Build history of the part. All positions in model axes, mm. A direction names the side the tool comes from. Coordinates: 2 decimals unless noted, no trailing zeros. Loops run counter-clockwise (first coordinate to the right, second up) from the corner with the lowest first, then second, coordinate; pieces in that order, holes last.
Item 1: Mould opens along Z. For faces 1 (the face through (6, 0, -1)), 2 (the face through (3.042, 14.012, 8.536)), 3 (the face through (2.949, 0.459, -34.887)), 4 (the face through (3, 0, -5)) say: released by +Z, released by -Z, zero draft, split by the parting line, or undercut.
Item 2: Cut at A-A (y = -14.5). List the corners of the cut face in (x, z), and give its area (3 significant figures).
Item 3: 3-axis set-ups, long thin cutter, end or side, ignore diameter. For faces 5 (the face through (0, 16, -42)), 6 (the face through (3, 0, -30)), 7 (the face through (0, -13, 1)), 8 (the face through (0, 16, 7)): which of +Z, -Z, +X, -X, +Y, -Y reach the whole face in a straight line?
Item 4: Flat gauge pins, fed straight in: pin 1 (2 mm diameter, centred on x = -6, y = -10, fed in from -Z); pin 2 (6.5 mm diameter, centred on y = 14.5, z = 4, fed in from +X); pin 3 (1 mm diameter, centred on x = -1, y = -14, fed in from +Z); pin 4 (3 mm diameter, centred on y = 4.5, z = -4, fed in from -X). Where does each tip first touch, or does it go through?
Item 5: Drill centre lines: line 1 along Y through (x, z) = (3.6, 4); line 2 along Y through (x, z) = (-13.5, -15); line 3 along Z through (x, y) = (-4.25, -4.5). Where is each one in solid material? Low to high.
from build123d import *

# Parameters (mm, degrees)
BOSS_EXTRUDE2_DEPTH      = 21.5
CUT_EXTRUDE8_DEPTH       = 44
CUT_EXTRUDE9_DEPTH       = 24.5
SKETCH18_R               = 2.5
CUT_EXTRUDE13_DEPTH      = 18.5000001
CUT_EXTRUDE13_DEPTH_BACK = 7.0000001
SKETCH19_RX              = 11.071840333
SKETCH19_RY              = 5.954349413
CUT_EXTRUDE14_DEPTH      = 7.0000001
CUT_EXTRUDE14_DEPTH_BACK = 18.5000001
FILLET6_R                = 2
FILLET7_R                = 2


with BuildPart() as part:
    # Sketch12 → Boss-Extrude2 (new body, symmetric)
    with BuildSketch(Plane(origin=(0, 0, 0), x_dir=(1, 0, 0), z_dir=(0, 1, 0))):
        with BuildLine():
            Line((0, 35), (0, 52))
            Line((0, 52), (6, 52))
            Line((6, 52), (6, -17))
            Line((6, -17), (0, -17))
            Line((0, -17), (0, 0))
            ThreePointArc((0, 0), (-17.5, 17.5), (0, 35))
        make_face()
    extrude(amount=BOSS_EXTRUDE2_DEPTH, both=True)

    # Sketch13 → Cut-Extrude8 (cut, through all)
    with BuildSketch(Plane.XZ.offset(21.5)):
        with BuildLine():
            Line((0, -30), (6, -30))
            Line((6, -30), (6, -5))
            Line((6, -5), (0, -5))
            ThreePointArc((0, -5), (-12.5, -17.5), (0, -30))
        make_face()
    extrude(amount=-CUT_EXTRUDE8_DEPTH, mode=Mode.SUBTRACT)

    # Sketch14 → Cut-Extrude9 (cut, through all)
    with BuildSketch(Plane(origin=(6, 0, 0), x_dir=(0, 0, -1), z_dir=(1, 0, 0))):
        with BuildLine():
            Line((-3.475, -21.5), (-17, -21.5))
            Line((-17, -21.5), (-17, 21.5))
            Line((-17, 21.5), (-5.475, 21.5))
            ThreePointArc((-5.475, 21.5), (-8.517618353, 13.892451617), (-3.272109233, 7.598251675))
            ThreePointArc((-3.272109233, 7.598251675), (0.112562803, 0.342782413), (-3.475, -6.814537766))
            ThreePointArc((-3.475, -6.814537766), (-8.299421353, -14.157268883), (-3.475, -21.5))
        make_face()
    cut_extrude9 = extrude(amount=-CUT_EXTRUDE9_DEPTH, mode=Mode.SUBTRACT)

    # Mirror1: Cut-Extrude9 across plane
    add(cut_extrude9.mirror(Plane.XY.offset(-17.5)), mode=Mode.SUBTRACT)

    # Sketch18 → Cut-Extrude13 (cut, two sides)
    with BuildSketch(Plane.ZY) as cut_extrude13_sk:
        with Locations((-39, 14.5)):
            Circle(SKETCH18_R)
        with Locations((4, 14.5)):
            Circle(SKETCH18_R)
        with Locations((-39, -14.5)):
            Circle(SKETCH18_R)
        with Locations((4, -14.5)):
            Circle(SKETCH18_R)
    extrude(amount=CUT_EXTRUDE13_DEPTH, mode=Mode.SUBTRACT)
    extrude(cut_extrude13_sk.sketch, amount=-CUT_EXTRUDE13_DEPTH_BACK, mode=Mode.SUBTRACT)

    # Sketch19 → Cut-Extrude14 (cut, two sides)
    with BuildSketch(Plane(origin=(0, 0, 0), x_dir=(0, 0, -1), z_dir=(1, 0, 0))) as cut_extrude14_sk:
        with Locations(Location((17.5, 0), (0, 0, 0))):
            Ellipse(SKETCH19_RX, SKETCH19_RY)
    extrude(amount=CUT_EXTRUDE14_DEPTH, mode=Mode.SUBTRACT)
    extrude(cut_extrude14_sk.sketch, amount=-CUT_EXTRUDE14_DEPTH_BACK, mode=Mode.SUBTRACT)

    # Fillet6
    fillet6_edges = [part.edges().sort_by_distance(p)[0] for p in [
        (0, 11.706035382, 0),
    ]]
    fillet(fillet6_edges, radius=FILLET6_R)

    # Fillet7
    fillet7_edges = [part.edges().sort_by_distance(p)[0] for p in [
        (0, 11.706035382, -35),
    ]]
    fillet(fillet7_edges, radius=FILLET7_R)


solid = part.part
Filled sheet:
1. face 1: zero draft
1. face 2: released by +Z
1. face 3: released by -Z
1. face 4: undercut
2. outline: (0, -43.29) - (6, -43.29) - (6, -41.5) - (0, -41.5) - close; (0, -36.5) - (6, -36.5) - (6, -30) - (0, -30) arc R12.5 cw to (0, -5) - (6, -5) - (6, 1.5) - (0, 1.5) - (0, 0) arc R17.5 ccw to (0, -35) - close; (0, 6.5) - (6, 6.5) - (6, 8.29) - (0, 8.29) - close
2. area: 335 mm2
3. face 5: -Z, -X, +Y, -Y
3. face 6: +X, +Y, -Y
3. face 7: +Z, -X, -Y
3. face 8: +Z, -X, +Y, -Y
4. pin 1: stops at z = -34.27
4. pin 2: stops at x = 6
4. pin 3: stops at z = -0.01
4. pin 4: stops at x = -12.74
5. line 1: y = -21.25 to -17, -12 to -7.06, 7.9 to 12, 17 to 21.5
5. line 2: y = -21.5 to -5.8, 5.8 to 21.5
5. line 3: z = -34.48 to -29.26, -5.74 to -0.52
